Autodesk Fusion 360 part; units mm, degrees
sketch "Sketch1" plane through (0, 0, 0) normal (0, 1, 0) x (1, 0, 0)
  line L0 (90, -90) -> (-90, -90)
  line L1 (-90, -90) -> (-90, 90)
  line L2 (-90, 90) -> (90, 90)
  line L3 (90, 90) -> (90, -90)
  line L4 (90, -90) -> (-90, 90) construction
  line L5 (-90, -90) -> (90, 90) construction
  dimension "d1" = 180
  dimension "d2" = 180
extrude "Extrude1" add sketch "Sketch1" along normal blind 10
sketch "Sketch2" plane through (0, 10, 0) normal (0, 1, 0) x (-1, 0, 0)
  line L0 (-90, -90) -> (90, -90)
  line L1 (90, -90) -> (90, 90)
  line L2 (90, 90) -> (-90, 90)
  line L3 (-90, 90) -> (-90, -90)
  circle A0 centre (0, 0) radius 70
  dimension "d5" = 140
extrude "Extrude2" add sketch "Sketch2" along normal blind 100 contours A0
sketch "Sketch3" plane through (0, 0, 0) normal (0, 0, 1) x (1, 0, 0)
  line L0 (40, 40) -> (-40, 40)
  line L1 (-40, 40) -> (-40, 80)
  line L2 (-40, 80) -> (40, 80)
  line L3 (40, 80) -> (40, 40)
  line L4 (40, 40) -> (-40, 80) construction
  line L5 (-40, 40) -> (40, 80) construction
  point P0 (0, 60)
  dimension "d8" = 80
  dimension "d9" = 40
  dimension "d10" = 60
extrude "Extrude3" add sketch "Sketch3" along normal blind 100
sketch "Sketch4" plane through (0, 110, 0) normal (0, 1, 0) x (-1, 0, 0)
  circle A0 centre (0, 0) radius 70
  circle A1 centre (0, 0) radius 65
  dimension "d13" = -5
extrude "Extrude4" cut sketch "Sketch4" against normal blind 3 contours A1
sketch "Sketch5" plane through (0, 10, 0) normal (0, 1, 0) x (-1, 0, 0)
  circle A0 centre (0, 0) radius 70
  line L0 (-90, -90) -> (90, -90)
  line L1 (90, -90) -> (90, 90)
  line L2 (90, 90) -> (-90, 90)
  line L3 (-90, 90) -> (-90, -90)
  point P0 (80, -80)
  point P1 (-80, -80)
  point P2 (-80, 80)
  point P3 (80, 80)
  dimension "d16" = 10
  dimension "d17" = 10
  dimension "d18" = 10
  dimension "d19" = 10
  dimension "d20" = 10
  dimension "d21" = 10
  dimension "d22" = 10
  dimension "d23" = 10
hole "Hole1" at (-80, 10, 80) at (80, 10, 80) at (80, 10, -80) at (-80, 10, -80) direction (0, -1, 0) diameter 5 depth 10 tip angle 118 counterbore diameter 10 counterbore depth 2
fillet "Fillet1" radius 10 8 edges at (-90, 5, 90) (90, 5, 90) (90, 5, -90) (-90, 5, -90) (-40, 80, 78.7228) (-40, 40, 78.7228) (40, 80, 78.7228) (40, 40, 78.7228)
fillet "Fillet2" radius 2 24 edges at (87.0711, 10, -87.0711) (0, 10, -90) (-87.0711, 10, -87.0711) (-90, 10, 0) (-87.0711, 10, 87.0711) (0, 10, 90) (87.0711, 10, 87.0711) (90, 10, 0) (36.9012, 77.2363, 59.4835) (40, 60, 57.4456) (36.9012, 42.7637, 59.4835) (0, 40, 70) (-36.9012, 42.7637, 59.4835) (-40, 60, 57.4456) (-36.9012, 77.2363, 59.4835) (0, 80, 70) (-37.0711, 77.0711, 100) (-40, 60, 100) (-37.0711, 42.9289, 100) (0, 40, 100) (37.0711, 42.9289, 100) (40, 60, 100) (37.0711, 77.0711, 100) (0, 80, 100)
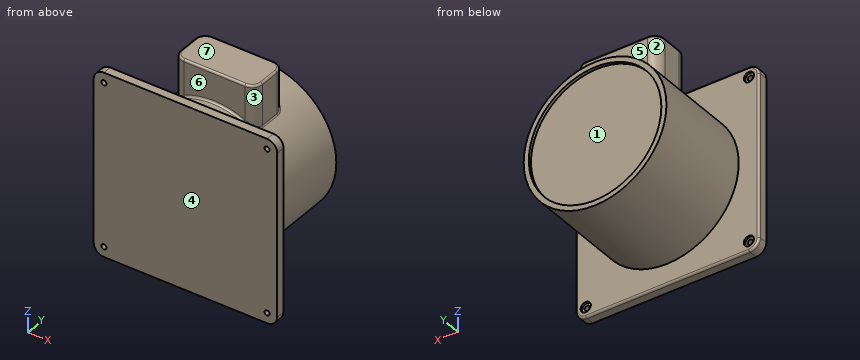
Design review of the part built by this model. Coordinates are the model's own, in mm. Face numbers are marked on the shaded views. A direction names the side the tool comes from. Round coordinates to 2 decimals unless told otherwise and drop trailing zeros. Loops run counter-clockwise (first coordinate to the right, second up) from the corner with the lowest first, then second, coordinate; pieces in that order, holes last. Notation, with made-up numbers: M -19,87 L 18,87 A18 cw 18,117 Z; hole C 78.25,-33.5 d6. An arc over 180 degrees is marked long. Answer as a JSON object with one key per item and string values.
Item 1: We need section A-A on z = 0. Give the boundary of the cut face in (x, y), and give its area (3 significant figures).
Answer sheet:
{"outline": "M -90,0 L 90,0 L 90,8 A2 ccw 88,10 L 70,10 L 70,110 L 65,110 L 65,107 L -65,107 L -65,110 L -70,110 L -70,10 L -88,10 A2 ccw -90,8 Z", "area": "15,400 mm^2"}
Item 2: We need section C-C on x = -54. Give the boundary of the cut face in (y, z).
Answer sheet:
{"outline": "M 0,-90 L 8,-90 A2 ccw 10,-88 L 10,-44.54 L 110,-44.54 L 110,-36.18 L 107,-36.18 L 107,36.18 L 110,36.18 L 110,44.54 L 10,44.54 L 10,88 A2 ccw 8,90 L 0,90 Z"}
Item 3: Wall thickness on L1, parallel to X at y = 5.5, z = -80; L2, parallel to Y at x = -8.5, z = 87: over which ranges is each line inside the solid? List them lowest first. Write a range as from..to.
Answer sheet:
{"L1": "x = -90..-82.5, -77.5..77.5, 82.5..90", "L2": "y = 0..10, 40..80"}
Item 4: Clearance check with flat-ended pins moving along their axes: P1, Ø22, axis at y = 63.5, z = 71, coming from the -X side; P2, Ø11, axis at x = 78, z = -79.5, coming from the +Y side; P3, Ø9, axis at x = -5, y = 2.5, coming from the +Z side. State where each tip first meets the part, or that it passes through.
Answer sheet:
{"P1": "stops at x = -40", "P2": "stops at y = 10", "P3": "stops at z = 90"}
Item 5: Machinability: for the marked faces 1, 2, 3 and 4, which of the approach directions +Z, -Z, +X, -X, +Y, -Y give a long, thin tool a straight path to every point of the face, cutting with its end or side? Answer none if there is none.
Answer sheet:
{"face 1": "+Y", "face 2": "+Z, -X, +Y", "face 3": "+Z, +X", "face 4": "+Z, -Z, +X, -X, -Y"}
Item 6: We need section B-B on x = 0. Give the boundary of the cut face in (y, z), and give its area (3 significant figures).
Answer sheet:
{"outline": "M 0,-90 L 8,-90 A2 ccw 10,-88 L 10,-70 L 110,-70 L 110,-65 L 107,-65 L 107,65 L 110,65 L 110,70 L 82,70 A2 cw 80,72 L 80,98 A2 ccw 78,100 L 42,100 A2 ccw 40,98 L 40,72 A2 cw 38,70 L 10,70 L 10,88 A2 ccw 8,90 L 0,90 Z", "area": "16,600 mm^2"}
Item 7: The part is to be moulded in two halves that separate along Y. For the marked faces 5, 6 and 7, say which applies: pulls with the +Y half, pulls with the -Y half, needs draft (parallel to the pull), parting line crosses it, or undercut.
Answer sheet:
{"face 5": "pulls with the +Y half", "face 6": "undercut", "face 7": "needs draft"}
